Study the drawing (mm; zero at the part's minimum x, y, z) and answer. Coordinates: 2 decimals unless noted, no trailing zeros. Loops run counter-clockwise (first coordinate to the right, second up) from the corner with the lowest first, then second, coordinate; pieces in that order, holes last. Notation, with made-up numbers: (36, 72.25) -> (40, 72.25) arc R31 cw to (40, 109.25) -> close; hole circle Ø7 at (-15, 83). An arc over 180 degrees is marked (long way). Answer as CSV lines item,"result".
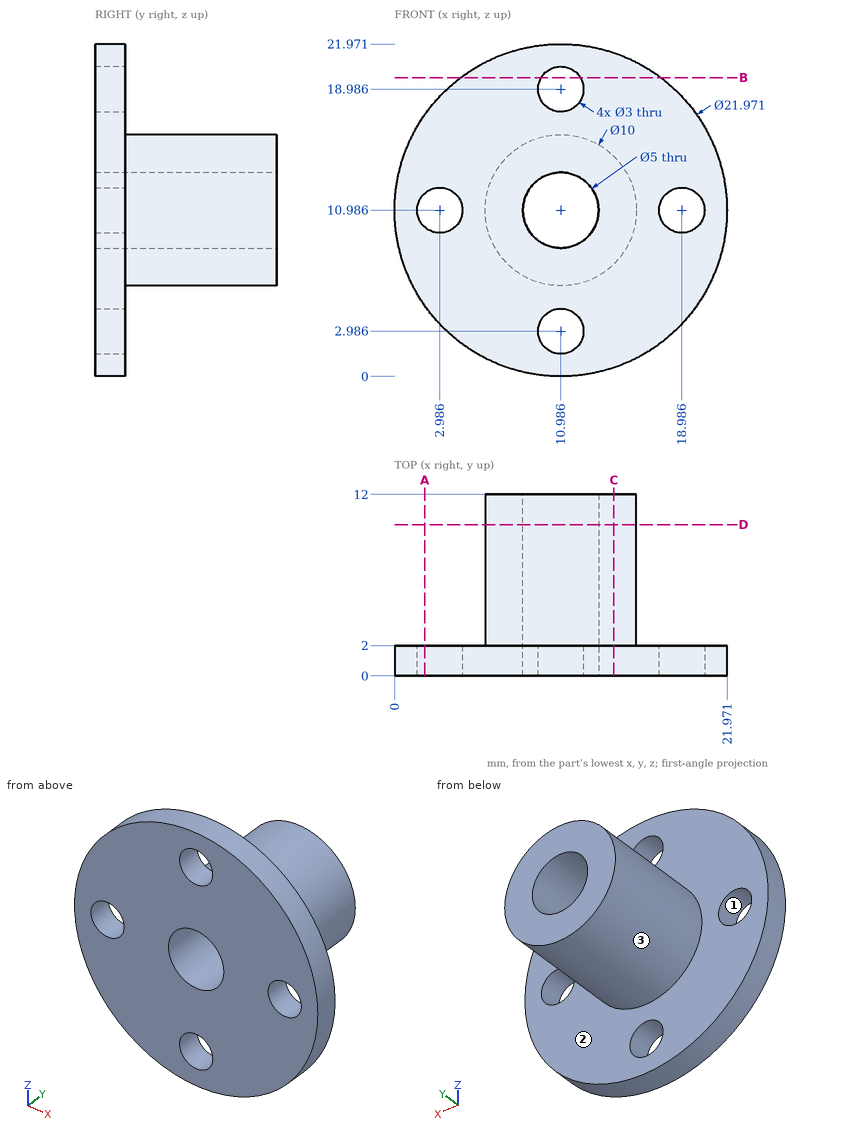
Q1. A cutting plane is placed at A-A, the plane x = 2. Write down the section's boundary in (y, z) (1 decimal).
Results:
outline,"(0, 4.7) -> (2, 4.7) -> (2, 9.9) -> (0, 9.9) -> close; (0, 12.1) -> (2, 12.1) -> (2, 17.3) -> (0, 17.3) -> close"
Q2. Given pin 1 Ø8 at (x, z) = (18.5, 4.5) entering from -Y; pin 2 Ø1 at (y, z) = (10, 14) entering from +X; pin 3 Ø3 at (x, y) = (16.5, 8) entering from +Z (1 decimal); pin 4 Ø8 at (x, z) = (4, 5) entering from +Y, each flat-ended and moving along its own axis, determine where each tip first touches the part or whether it passes through.
Results:
pin 1,"stops at y = 0"
pin 2,"stops at x = 15.31"
pin 3,"stops at z = 14"
pin 4,"stops at y = 2"
Q3. For a pull along X with two mould halves and no side action, classify the marked faces 1, 2 and 3 as pulls with the +X half, pulls with the -X half, needs draft (parallel to the pull), parting line crosses it, or undercut.
Results:
face 1,"undercut"
face 2,"needs draft"
face 3,"parting line crosses it"
Q4. A cutting plane is placed at D-D, the plane y = 10. Write down the section's boundary in (x, z) (1 decimal).
Results:
outline,"circle Ø10 at (11, 11); hole circle Ø5 at (11, 11)"
Q5. A cutting plane is placed at B-B, the plane z = 19.75. Write down the section's boundary in (x, y) (1 decimal).
Results:
outline,"(4.4, 0) -> (9.7, 0) -> (9.7, 2) -> (4.4, 2) -> close; (12.3, 0) -> (17.6, 0) -> (17.6, 2) -> (12.3, 2) -> close"
Q6. Find the intervals of material crossed by probe 1 along X at (y, z) = (4.5, 11) (1 decimal); probe 2 along X at (y, z) = (1.5, 11.5) (1 decimal); probe 3 along Y at (x, z) = (18, 19), in increasing order. Write a range as [from, to].
Results:
probe 1,"x = [6, 8.5], [13.5, 16]"
probe 2,"x = [0, 1.6], [4.4, 8.5], [13.4, 17.6], [20.4, 22]"
probe 3,"y = [0, 2]"
Q7. A cutting plane is placed at C-C, the plane x = 14.5. Write down the section's boundary in (y, z).
Results:
outline,"(0, 0.58) -> (2, 0.58) -> (2, 7.43) -> (12, 7.43) -> (12, 14.54) -> (2, 14.54) -> (2, 21.39) -> (0, 21.39) -> close"
